from build123d import *

# Parameters (mm, degrees)
SKETCH_1_W          = 7.5
SKETCH_1_H          = 6
EXTRUDE_1_DEPTH     = 2
SKETCH_2_W          = 12.9
SKETCH_2_H          = 3.9
EXTRUDE_2_DEPTH     = 52
SKETCH_3_R          = 1.6
CUT_EXTRUDE_1_DEPTH = 356
SKETCH_4_W          = 7.5
SKETCH_4_H          = 1.05
CUT_EXTRUDE_2_DEPTH = 10
SKETCH_5_W          = 22.28550744
SKETCH_5_H          = 23.147494016
CUT_EXTRUDE_3_DEPTH = 10


with BuildPart() as part:
    # 草图1 → 凸台-拉伸1 (new body)
    with BuildSketch(Plane.XY):
        with Locations((3.75, 0)):
            Rectangle(SKETCH_1_W, SKETCH_1_H)
    extrude(amount=EXTRUDE_1_DEPTH)

    # 草图2 → 凸台-拉伸2 (add)
    with BuildSketch(Plane.XY.offset(2)):
        Rectangle(SKETCH_2_W, SKETCH_2_H)
    extrude(amount=EXTRUDE_2_DEPTH)

    # 草图3 → 切除-拉伸1 (cut)
    with BuildSketch(Plane.XZ.offset(1.95)):
        with Locations((3.5, 37)):
            Circle(SKETCH_3_R)
        with Locations((3.5, 11)):
            Circle(SKETCH_3_R)
        with Locations((-3.5, 24)):
            Circle(SKETCH_3_R)
        with Locations((0, 50)):
            Circle(SKETCH_3_R)
    extrude(amount=-CUT_EXTRUDE_1_DEPTH, mode=Mode.SUBTRACT)

    # 草图4 → 切除-拉伸2 (cut)
    with BuildSketch(Plane.XY.offset(2)):
        with Locations((3.75, 2.475)):
            Rectangle(SKETCH_4_W, SKETCH_4_H)
    extrude(amount=-CUT_EXTRUDE_2_DEPTH, mode=Mode.SUBTRACT)

    # 草图5 → 切除-拉伸3 (cut)
    with BuildSketch(Plane(origin=(0, 1.95, 0), x_dir=(1, 0, 0), z_dir=(0, 1, 0))):
        with Locations((0, 4.573747008)):
            Rectangle(SKETCH_5_W, SKETCH_5_H)
    extrude(amount=-CUT_EXTRUDE_3_DEPTH, mode=Mode.SUBTRACT)


solid = part.part
Input: part model. Units: mm. Frame: model coordinates. Round coordinates to 2 decimals unless told otherwise and drop trailing zeros. Order: outer loops, then holes, each group sorted by start corner. A loop starts at its lowest first (then second) coordinate and runs counter-clockwise, first axis right, second up. Notation, with made-up numbers: (45.25, 21) - (97.25, 21) arc R23 ccw to (97.25, 40) - close; hole circle Ø1 at (-14, 76.5). An arc over 180 degrees is marked (long way). Answer as a JSON object with one key per item and string values. Group by question number.
(1) Draft query along Z for faces 1 (the face through (-6.45, 0, 30)), 2 (the face through (0, 0, 54)), 3 (the face through (0.86, -0.03, 51.35)). Return one class per face: released by +Z, released by -Z, zero draft, split by the parting line, or undercut.
(2) Cut plane C-C (x = -3.5). Return loops of the section in (y, z).
(3) Cut plane D-D (x = 4). Return loops of the section in (y, z), then the cut area to 3 significant figures.
(4) Cut plane A-A (z = 24). Return loops of the section in (x, y).
(5) Material intervals for probe 1 along Z at (x, y) = (3.5, 0.6); probe 2 along Z at (x, y) = (0, 0.9); probe 3 along Z at (x, y) = (-3.5, -0.95), sorted ascending. Write a range as from..to.
(6) Cut plane B-B (y = -1.4). Return loops of the section in (x, z).
Here are the results:
{
 "1": {"face 1": "zero draft", "face 2": "released by +Z", "face 3": "undercut"},
 "2": {"outline": "(-1.95, 7) - (1.95, 7) - (1.95, 22.4) - (-1.95, 22.4) - close; (-1.95, 25.6) - (1.95, 25.6) - (1.95, 54) - (-1.95, 54) - close"},
 "3": {"outline": "(-1.95, 7) - (1.95, 7) - (1.95, 9.48) - (-1.95, 9.48) - close; (-1.95, 12.52) - (1.95, 12.52) - (1.95, 35.48) - (-1.95, 35.48) - close; (-1.95, 38.52) - (1.95, 38.52) - (1.95, 54) - (-1.95, 54) - close", "area": "160 mm^2"},
 "4": {"outline": "(-6.45, -1.95) - (-5.1, -1.95) - (-5.1, 1.95) - (-6.45, 1.95) - close; (-1.9, -1.95) - (6.45, -1.95) - (6.45, 1.95) - (-1.9, 1.95) - close"},
 "5": {"probe 1": "z = 7..9.4, 12.6..35.4, 38.6..54", "probe 2": "z = 7..48.4, 51.6..54", "probe 3": "z = 7..22.4, 25.6..54"},
 "6": {"outline": "(-6.45, 7) - (6.45, 7) - (6.45, 54) - (-6.45, 54) - close; hole circle Ø3.2 at (-3.5, 24); hole circle Ø3.2 at (0, 50); hole circle Ø3.2 at (3.5, 11); hole circle Ø3.2 at (3.5, 37)"}
}
